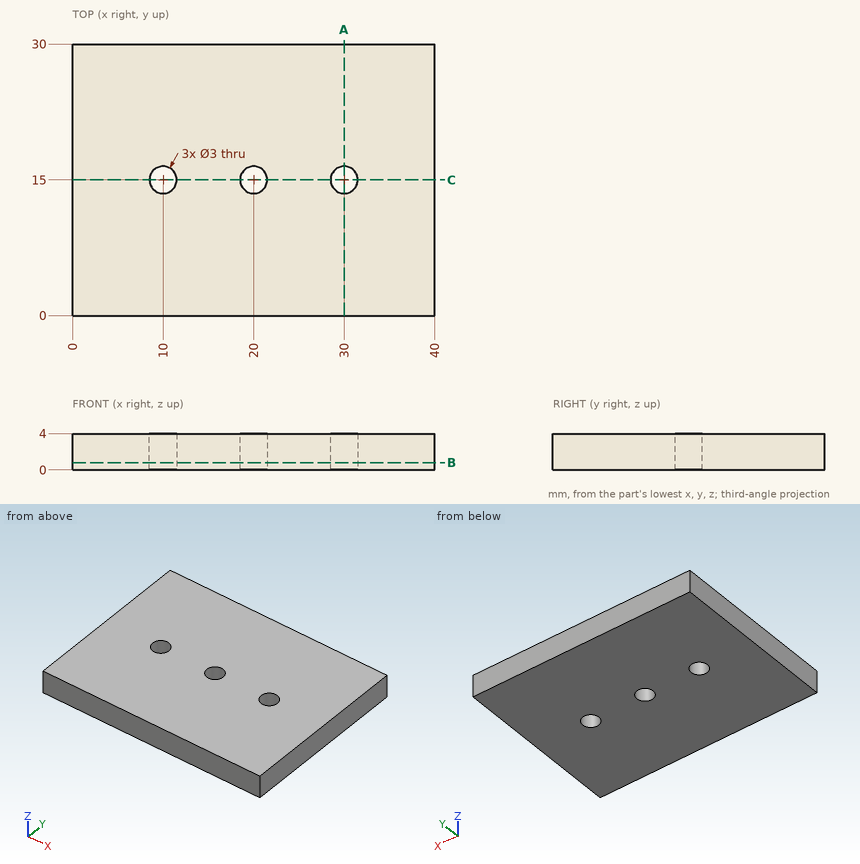
Can you work these out from the drawing? Everything is in mm from the part's minimum corner. Give positions to 0.01 mm unless a question says otherwise; leave off trailing zeros. Loops run counter-clockwise (first coordinate to the right, second up) from the corner with the lowest first, then second, coordinate; pieces in that order, holes last. Notation, with made-up numbers: (76.5, -4.5) -> (122.5, -4.5) arc R12 ccw to (122.5, 2.5) -> close; hole circle Ø10 at (20.25, 26). An arc over 180 degrees is marked (long way). Return JSON: item names as keys, results as strings.
Item 1: If we section it at C-C on y = 15: List the corners of the cut face in (x, z) for me, plus the area to 3 significant figures.
Geometry results:
{"outline": "(0, 0) -> (8.5, 0) -> (8.5, 4) -> (0, 4) -> close; (11.5, 0) -> (18.5, 0) -> (18.5, 4) -> (11.5, 4) -> close; (21.5, 0) -> (28.5, 0) -> (28.5, 4) -> (21.5, 4) -> close; (31.5, 0) -> (40, 0) -> (40, 4) -> (31.5, 4) -> close", "area": "124 mm²"}
Item 2: I'm going to push a flat-ended pin straight in: pin 1 (1.8 mm diameter, centred on x = 10, y = 15, fed in from -Z). Where does the tip first touch, or does it pass through?
Geometry results:
{"pin 1": "passes through"}
Item 3: If we section it at B-B on z = 0.8: List the corners of the cut face in (x, y) for me.
Geometry results:
{"outline": "(0, 0) -> (40, 0) -> (40, 30) -> (0, 30) -> close; hole circle Ø3 at (10, 15); hole circle Ø3 at (20, 15); hole circle Ø3 at (30, 15)"}
Item 4: I need wall thicknesses on L1, parallel to Y at x = 10, z = 2.7; L2, parallel to X at y = 13.75, z = 3.3; L3, parallel to X at y = 14.25, z = 0.65. Which ranges of each line are inside material? Lowest first, please. Write a range as from..to.
Geometry results:
{"L1": "y = 0..13.5, 16.5..30", "L2": "x = 0..9.17, 10.83..19.17, 20.83..29.17, 30.83..40", "L3": "x = 0..8.7, 11.3..18.7, 21.3..28.7, 31.3..40"}
Item 5: If we section it at A-A on x = 30: List the corners of the cut face in (y, z) for me, plus the area to 3 significant figures.
Geometry results:
{"outline": "(0, 0) -> (13.5, 0) -> (13.5, 4) -> (0, 4) -> close; (16.5, 0) -> (30, 0) -> (30, 4) -> (16.5, 4) -> close", "area": "108 mm²"}
